```python
from build123d import *

# Parameters (mm, degrees)
CUT_EXTRUDE_START   = 5
SKETCH_2_W          = 25
SKETCH_2_H          = 23.22226429
CUT_EXTRUDE_1_DEPTH = 23.156951228
HOLE_WIZARD_M5_1_D  = 4.2


with BuildPart() as part:
    # 草图1 → 旋转1 (revolve)
    with BuildSketch(Plane.XY, mode=Mode.PRIVATE) as revolve_1_sk:
        Polygon((0, 7.5), (12.5, 7.5), (12.5, 5), (25, 5), (25, 0), (0, 0), align=None)
    revolve_1 = revolve(revolve_1_sk.sketch.rotate(Axis((0, 0, 0), (1, 0, 0)), 90), axis=Axis((0, 0, 0), (1, 0, 0)))

    # 镜向1: 旋转1 across plane
    add(revolve_1.mirror(Plane(origin=(0, 0, 0), x_dir=(0, 0, 1), z_dir=(1, 0, 0))))

    # 草图2 → 切除-拉伸1 (cut, through all)
    with BuildSketch(Plane(origin=(0, 0, 0), x_dir=(1, 0, 0), z_dir=(0, 1, 0)).offset(CUT_EXTRUDE_START)):
        Rectangle(SKETCH_2_W, SKETCH_2_H)
    extrude(amount=CUT_EXTRUDE_1_DEPTH, mode=Mode.SUBTRACT)

    # M5 螺纹孔的螺纹孔钻头1 (through all)
    with Locations(Plane(origin=(0, 5, 0), x_dir=(1, 0, 0), z_dir=(0, 1, 0))):
        with Locations((0, 0)):
            Hole(HOLE_WIZARD_M5_1_D / 2)


solid = part.part
```
Geometry check sheet. Reference: the model listing, model coordinates, mm. A direction names the side the tool comes from. Give positions to 0.01 mm unless a question says otherwise; leave off trailing zeros. Loops run counter-clockwise (first coordinate to the right, second up) from the corner with the lowest first, then second, coordinate; pieces in that order, holes last. Notation, with made-up numbers: M 37.5,77 L 86.5,77 A34 cw 86.5,112 Z; hole C 77,80 d2. An arc over 180 degrees is marked long. Write item = value, one per line.
(1) Gauge pin test, flat ends, axial feed: pin 1 Ø4 at (x, y) = (-17.5, 3) entering from -Z; pin 2 Ø3 at (x, z) = (-19, 3.5) entering from -Y; pin 3 Ø2 at (x, y) = (9.5, -4) entering from +Z. Record the tip position at first contact, or that the pin passes through.
Answer below:
pin_1 = -4.9
pin_2 = -4.58
pin_3 = 6.87
(2) Release check for a two-part mould opening along X. For faces 1 (the face through (0, 5, -3)), 2 (the face through (-2.003, -1.341, -0.631)), 3 (the face through (-25, 0, 0)) record: released by +X, released by -X, zero draft, split by the parting line, or undercut.
Answer below:
face_1 = zero draft
face_2 = undercut
face_3 = released by -X
(3) Sectioned sample at D-D, the plane x = 9.5. Record the cut outline in (y, z).
Answer below:
outline = M 5,-5.59 L 5,5.59 A7.5 ccw long Z
(4) Tool access check on faces 4 (the face through (-0.18, -6.42, 3.88)), 5 (the face through (19, 0, -5)), 6 (the face through (-12.5, -6, 0)). Record the directions out of +Z, -Z, +X, -X, +Y, -Y that give a thin tool (end or side, any length) a straight path to the whole face; none if there is none.
Answer below:
face_4 = +X, -X
face_5 = +X
face_6 = -X
(5) Sectioned sample at A-A, the plane x = 0. Record the cut outline in (y, z).
Answer below:
outline = M -7.2,-2.1 A7.5 ccw 5,-5.59 L 5,-2.1 Z; M -7.2,2.1 L 5,2.1 L 5,5.59 A7.5 ccw Z
(6) Sectioned sample at B-B, the plane y = 0. Record the cut outline in (x, z).
Answer below:
outline = M -25,-5 L -12.5,-5 L -12.5,-7.5 L 12.5,-7.5 L 12.5,-5 L 25,-5 L 25,5 L 12.5,5 L 12.5,7.5 L -12.5,7.5 L -12.5,5 L -25,5 Z; hole C 0,0 d4.2
(7) Material ranges on line 1 (Z direction, x = 0, y = -0.25); line 2 (Z direction, x = 0, y = -3.5); line 3 (X direction, y = 3.5, z = -6.25), recorded low to high. Write a range as [from, to].
Answer below:
line_1 = [-7.5, -2.1], [2.1, 7.5]
line_2 = [-6.63, -2.1], [2.1, 6.63]
line_3 = [-12.5, 12.5]
